For this review, take the finished solid that the model builds, in its own axes (mm). Face numbers are marked on the shaded views. A direction names the side the tool comes from. Give positions to 0.01 mm unless a question says otherwise; leave off trailing zeros. Write each loop counter-clockwise with the first axis right and the second up, starting at its lowest first coordinate (ties: lowest second). Pieces come first, ordered by that corner, then holes. Notation, with made-up numbers: (72.5, 17.25) -> (121.5, 17.25) arc R26 cw to (121.5, 31.25) -> close; hole circle Ø11 at (71.25, 0). An arc over 180 degrees is marked (long way). Answer as CSV lines item,"result".
Autodesk Inventor part; units mm, degrees
ref_plane "YZ Plane" through (0, 0, 0) normal (1, 0, 0) x (0, 1, 0)
ref_plane "XZ Plane" through (0, 0, 0) normal (0, 1, 0) x (-1, 0, 0)
ref_plane "XY Plane" through (0, 0, 0) normal (0, 0, 1) x (1, 0, 0)
sketch "Sketch1" plane through (0, 0, 0) normal (0, 0, 1) x (1, 0, 0)
  circle A0 centre (0, 0) radius 12.7
  circle A1 centre (0, 0) radius 14.2875
  line L0 (-5.2917, 5.9163) -> (5.2917, 5.9163)
  line L1 (5.2917, 5.9163) -> (5.2917, -5.9163)
  line L2 (5.2917, -5.9163) -> (-5.2917, -5.9163)
  line L3 (-5.2917, -5.9163) -> (-5.2917, 5.9163)
  arc A2 (5.2917, 5.9163) -> (-5.2917, 5.9163) centre (0, 0) ccw
  arc A3 (-5.2917, -5.9163) -> (5.2917, -5.9163) centre (0, 0) ccw
  dimension "d2" = 25.4
  dimension "d3" = 28.575
  dimension "d4" = 10.5833
  dimension "d5" = 5.2917
  dimension "d6" = 11.8325
  dimension "d7" = 5.9163
  dimension "d8" = 7.9375
extrude "Extrusion1" add sketch "Sketch1" against normal blind 200.025 contours A1
fillet "Fillet1" radius 0.7937 2 edges at (-14.2875, 0, 0) (-14.2875, 0, -200.025)
extrude "Extrusion2" add sketch "Sketch1" along normal blind 12.7 contours A0 | A1
extrude "Extrusion3" add sketch "Sketch1" along normal blind 28.575 contours A2 L0 | L0 L1 L2 L3 | L2 A3
chamfer "Chamfer1" distance 1.5875 angle 45 1 edges at (-14.2875, 0, 12.7)
thread "Thread1"
thread "Thread2"
sketch "Sketch2" plane through (0, 0, -200.025) normal (0, 0, -1) x (-1, 0, 0)
  circle A0 centre (0, 0) radius 14.2875
  circle A1 centre (0, 0) radius 7.9375
  circle A2 centre (0, 0) radius 3.175
  circle A3 centre (0, 0) radius 3.9688
  dimension "d24" = 15.875
  dimension "d25" = 7.9375
  dimension "d26" = 6.35
extrude "Extrusion4" add sketch "Sketch2" along normal blind 12.7 contours A0
extrude "Extrusion5" add sketch "Sketch2" along normal blind 19.05 contours A3
fillet "Fillet2" radius 0.1905 2 edges at (3.9688, 0, -219.075) (3.175, 0, -219.075)
extrude "Extrusion6" add sketch "Sketch2" along normal blind 31.75 contours A1
chamfer "Chamfer2" distance 1.5875 angle 45 1 edges at (14.2875, 0, -212.725)
thread "Thread3"
sketch "Sketch3" plane through (5.2917, -5.9163, 12.7) normal (1, 0, 0) x (0, 0, -1)
  line L0 (0, 11.8325) -> (-15.875, 11.8325)
  line L1 (-15.875, 11.8325) -> (-15.875, 0)
  line L2 (0, 0) -> (-15.875, 0)
  circle A0 centre (-9.525, 5.9163) radius 3.175
  point P0 (12.7, 5.9163)
  dimension "d39" = 6.35
  dimension "d40" = 5.9163
  dimension "d41" = 11.8325
  dimension "d42" = 6.35
extrude "Extrusion7" cut sketch "Sketch3" against normal blind 25.4
equation "\"d40\" = 0.5 * d41"
properties part number "6''  by 1'' dia piston"
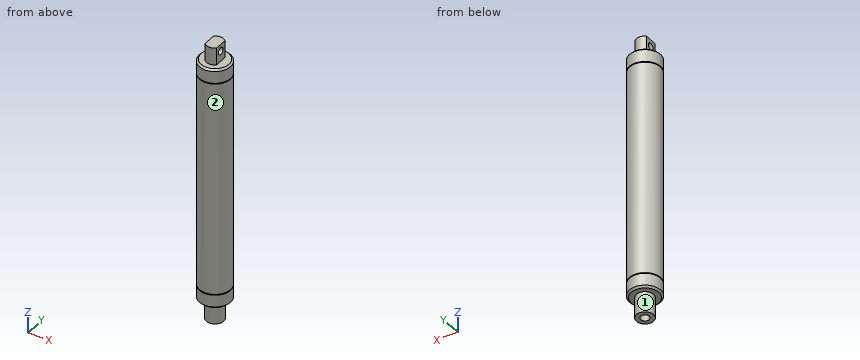
Q1. For the marked faces 1 and 2, list the 3-axis set-ups (+Z, -Z, +X, -X, +Y, -Y) from which the entire face can be reached by the end or side of a thin tool; tool diameter is ignored.
Answer block:
face 1,"-Z"
face 2,"+Z, -Z"
Q2. Clearance check with flat-ended pins moving along their axes: pin 1 (1 mm diameter, centred on x = 1, y = -10, fed in from -Z) (3 decimals); pin 2 (3.5 mm diameter, centred on y = -2.5, z = 24, fed in from +X); pin 3 (6 mm diameter, centred on x = 2.5, y = 11.5, fed in from +Z). State where each tip first meets the part, or that it passes through.
Answer block:
pin 1,"stops at z = -212.725"
pin 2,"stops at x = 5.29"
pin 3,"stops at z = 12.7"
Q3. To check wall thickness, follow probe 1 along Y at (x, z) = (0, -224); probe 2 along Z at (x, y) = (-5.25, 11) (3 decimals); probe 3 along Z at (x, y) = (-6.5, -3.25) (3 decimals). State the ranges of each line that lie inside material, in increasing order. Write a range as [from, to].
Answer block:
probe 1,"y = [-7.94, -3.97], [3.97, 7.94]"
probe 2,"z = [-212.725, -200.025], [0, 12.7]"
probe 3,"z = [-231.775, -200.025], [0, 12.7]"
Q4. Add section A-A (z = -71). Write out the cut boundary in (x, y) (1 decimal), plus the area to 3 significant figures.
Answer block:
outline,"circle Ø28.6 at (0, 0); hole circle Ø25.4 at (0, 0)"
area,"135 mm2"
